Job drawing, mm, ordinate dimensions from the low corner. One solid piece. Round coordinates to 2 decimals unless told otherwise and drop trailing zeros. Loops run counter-clockwise (first coordinate to the right, second up) from the corner with the lowest first, then second, coordinate; pieces in that order, holes last. Notation, with made-up numbers: M 50.25,29.5 L 70.25,29.5 A29 ccw 70.25,65.5 Z; hole C 38.5,85.5 d4. An arc over 180 degrees is marked long. One line per item, written item: value.
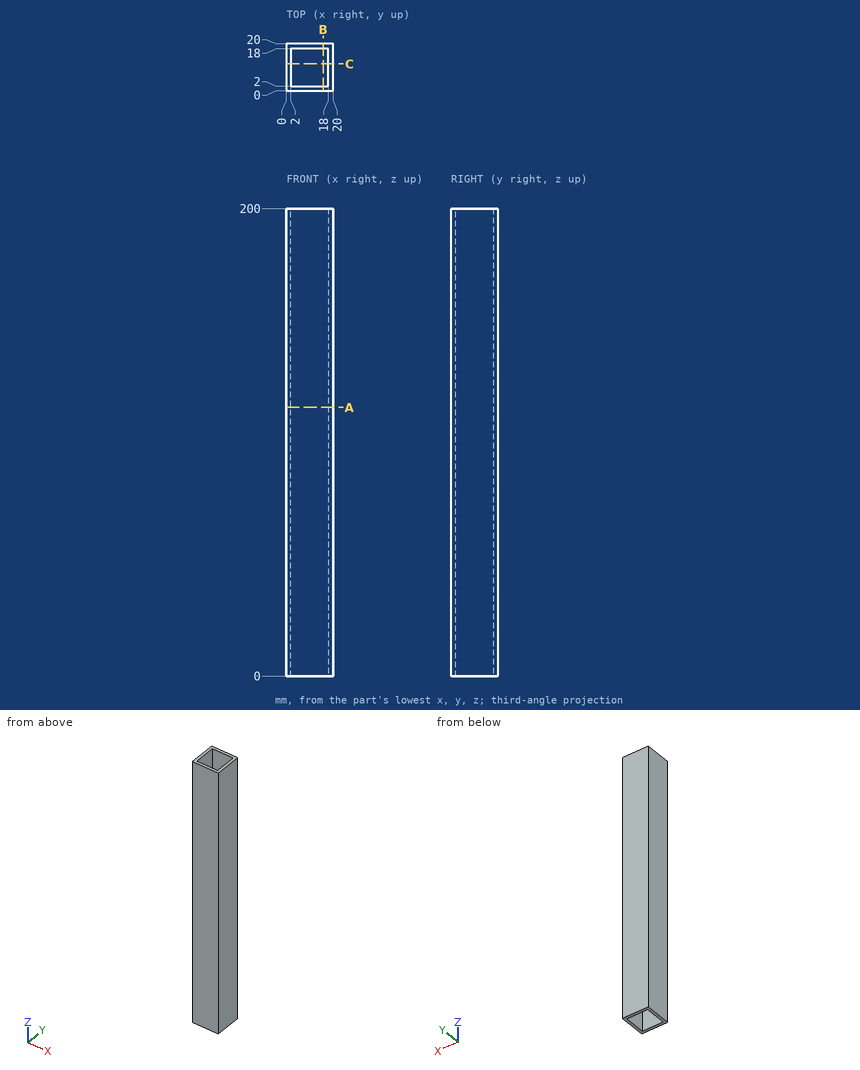
Item 1: Slice it at A-A, the plane z = 115. Give the cut face in (x, y), and give its area (3 significant figures).
Check values:
outline: M 0,0 L 20,0 L 20,20 L 0,20 Z; hole M 2,2 L 18,2 L 18,18 L 2,18 Z
area: 144 mm2
Item 2: Wall check: line 1 along Y through (x, z) = (8.25, 187.5). Give the ranges that are in metal, low to high.
Check values:
line 1: y = 0 to 2, 18 to 20
Item 3: Drop a flat-ended pin along its axis: P1, Ø8, axis at x = 6.5, y = 6.5, coming from the +Z side. Give the stop position or say it passes through.
Check values:
P1: passes through
Item 4: Slice it at B-B, the plane x = 15.75. Give the cut face in (y, z), and give its area (3 significant figures).
Check values:
outline: M 0,0 L 2,0 L 2,200 L 0,200 Z; M 18,0 L 20,0 L 20,200 L 18,200 Z
area: 800 mm2
